from build123d import *

# Parameters (mm, degrees)
SKIZZE1_W       = 10
SKIZZE1_H       = 3.5
ROTATION1_ANGLE = 270
VERRUNDUNG1_R   = 1.5
VERRUNDUNG2_R   = 0.8


with BuildPart() as part:
    # Skizze1 → Rotation1 (revolve, symmetric)
    with BuildSketch(Plane.XY) as rotation1_sk:
        with Locations((0, 15.25)):
            Rectangle(SKIZZE1_W, SKIZZE1_H)
    revolve(axis=Axis((-29.230918038, 0, 0), (1, 0, 0)), revolution_arc=ROTATION1_ANGLE / 2)
    revolve(rotation1_sk.sketch, axis=Axis((-29.230918038, 0, 0), (-1, 0, 0)), revolution_arc=ROTATION1_ANGLE / 2)

    # Verrundung1
    verrundung1_edges = [part.edges().sort_by_distance(p)[0] for p in [
        (0, -9.545941546, 9.545941546),
        (0, -12.02081528, -12.02081528),
        (0, -9.545941546, -9.545941546),
        (0, -12.02081528, 12.02081528),
    ]]
    fillet(verrundung1_edges, radius=VERRUNDUNG1_R)

    # Verrundung2
    verrundung2_edges = [part.edges().sort_by_distance(p)[0] for p in [
        (5, 17, 0),
        (-5, 17, 0),
        (-5, -10.731073787, -10.731073787),
        (-5, 13.5, 0),
        (-5, -10.731073787, 10.731073787),
        (-5, -11.346290795, 12.042038249),
        (-5, -9.56786945, 10.115976522),
        (-5, -9.56786945, -10.115976522),
        (-5, -11.346290795, -12.042038249),
        (5, -10.731073787, -10.731073787),
        (5, 13.5, 0),
        (5, -10.731073787, 10.731073787),
        (5, -11.346290795, 12.042038249),
        (5, -9.56786945, 10.115976522),
        (5, -9.56786945, -10.115976522),
        (5, -11.346290795, -12.042038249),
    ]]
    fillet(verrundung2_edges, radius=VERRUNDUNG2_R)


solid = part.part
Work out the finished part from the listing and answer in its coordinate system (mm). A direction names the side the tool comes from. Give positions to 0.01 mm unless a question says otherwise; leave off trailing zeros. Loops run counter-clockwise (first coordinate to the right, second up) from the corner with the lowest first, then second, coordinate; pieces in that order, holes last. Notation, with made-up numbers: (69, 22.5) - (77, 22.5) arc R5 cw to (77, 29.5) - close; hole circle Ø5 at (-35.75, 6). An arc over 180 degrees is marked (long way). Answer in a Markdown table with one row per item. Add a question column.
Q1. The part is cut by section C-C (x = 2.5). Determine the outline of the cut face in (y, z).
Q2. The part is cut by section B-B (z = 0). Determine the outline of the cut face in (x, y).
Q3. Each of these flat-tipped pins is pushed along its axis until it touches: P1, Ø6, axis at x = 1, y = 9.5, coming from the +Z side; P2, Ø1, axis at x = 3.5, z = -4, coming from the +Y side; P3, Ø5, axis at x = 2.5, z = -4, coming from the +Y side. Where does it stop, or does it pass through?
Q4. Determine the mould class of faces 4 (the flat face through (-5, 15, 0)), 5 (the cylindrical face through (-4.77, -10.56, 10.9)), 6 (the cylindrical face through (0.06, 16.99, 0.54)) for opening direction Z: released by +Z, released by -Z, zero draft, split by the parting line, or undercut.
Q5. The part is cut by section A-A (y = 0). Determine the outline of the cut face in (x, z).
Q6. Consider line 1 along Z through (x, y) = (-2, 0); line 2 along Y through (x, z) = (-0.5, 0); line 3 along Z through (x, y) = (2.75, 6). Determine where each line is inside the solid, lowest interval first.
Q7. A tool of negligible diameter and unlimited length cuts with its end or side. For faces 1 (the cylindrical face through (-4.77, -10.56, -10.9)), 2 (the cylindrical face through (0.059, -9.583, 10.117)), 3 (the cylindrical face through (4.76, -10.57, -10.89)), from which of +Z, -Z, +X, -X, +Y, -Y can it reach the whole face along a straight path? Write none if from no direction.
Solution:
| question | item | result |
|---|---|---|
| 1 | outline | (-10.91, -10.91) arc R1.5 ccw to (-10.8, -13.13) arc R17 ccw (long way) to (-10.8, 13.13) arc R1.5 ccw to (-10.91, 10.91) - (-10.55, 10.55) arc R1.5 ccw to (-8.54, 10.45) arc R13.5 cw (long way) to (-8.54, -10.45) arc R1.5 ccw to (-10.55, -10.55) - close |
| 2 | outline | (-5, 14.3) arc R0.8 ccw to (-4.2, 13.5) - (4.2, 13.5) arc R0.8 ccw to (5, 14.3) - (5, 16.2) arc R0.8 ccw to (4.2, 17) - (-4.2, 17) arc R0.8 ccw to (-5, 16.2) - close |
| 3 | P1 | stops at z = 15.71 |
| 3 | P2 | stops at y = 16.64 |
| 3 | P3 | stops at y = 16.93 |
| 4 | face 4 | zero draft |
| 4 | face 5 | undercut |
| 4 | face 6 | split by the parting line |
| 5 | outline | (-5, -16.2) arc R0.8 ccw to (-4.2, -17) - (4.2, -17) arc R0.8 ccw to (5, -16.2) - (5, -14.3) arc R0.8 ccw to (4.2, -13.5) - (-4.2, -13.5) arc R0.8 ccw to (-5, -14.3) - close; (-5, 14.3) arc R0.8 ccw to (-4.2, 13.5) - (4.2, 13.5) arc R0.8 ccw to (5, 14.3) - (5, 16.2) arc R0.8 ccw to (4.2, 17) - (-4.2, 17) arc R0.8 ccw to (-5, 16.2) - close |
| 6 | line 1 | z = -17 to -13.5, 13.5 to 17 |
| 6 | line 2 | y = 13.5 to 17 |
| 6 | line 3 | z = -15.91 to -12.09, 12.09 to 15.91 |
| 7 | face 1 | -X, -Y |
| 7 | face 2 | +X, -X |
| 7 | face 3 | +X, -Y |
